```python
from build123d import *

# Parameters (mm, degrees)
CROQUIS1_W              = 210
CROQUIS1_H              = 50
CROQUIS1_R              = 2.5
CROQUIS1_R_2            = 2
SALIENTE_EXTRUIR1_DEPTH = 10
REDONDEO1_R             = 20


with BuildPart() as part:
    # Croquis1 → Saliente-Extruir1 (new body)
    with BuildSketch(Plane.XY):
        with Locations((105, -25)):
            Rectangle(CROQUIS1_W, CROQUIS1_H)
        with Locations((96, -28)):
            Circle(CROQUIS1_R, mode=Mode.SUBTRACT)
        Polygon((118, -27), (123, -27), (123, -32), (123, -37), (118, -37), (92, -37), (87, -37), (87, -32), (87, -27), (92, -27), (92, -32), (118, -32), align=None, mode=Mode.SUBTRACT)
        with Locations((114, -28)):
            Circle(CROQUIS1_R, mode=Mode.SUBTRACT)
        with Locations((4, -25)):
            Circle(CROQUIS1_R_2, mode=Mode.SUBTRACT)
        Polygon((67, -12), (76, -12), (76, -17), (67, -17), (67, -32), (76, -32), (76, -37), (67, -37), (61, -37), (61, -32), (61, -17), (61, -12), align=None, mode=Mode.SUBTRACT)
        Polygon((138, -12), (148, -12), (148, -17), (138, -17), (138, -21.5), (143, -21.5), (148, -21.5), (148, -26.5), (148, -31), (148, -36), (133, -36), (133, -31), (143, -31), (143, -26.5), (138, -26.5), (133, -26.5), (133, -21.5), (133, -17), (133, -12), align=None, mode=Mode.SUBTRACT)
        Polygon((87, -18), (87, -13), (92, -13), (102.5, -13), (102.5, -6), (107.5, -6), (107.5, -13), (118, -13), (123, -13), (123, -18), (123, -23), (118, -23), (118, -18), (107.5, -18), (102.5, -18), (92, -18), (92, -23), (87, -23), align=None, mode=Mode.SUBTRACT)
        with Locations((206, -25)):
            Circle(CROQUIS1_R_2, mode=Mode.SUBTRACT)
    extrude(amount=SALIENTE_EXTRUIR1_DEPTH)

    # Redondeo1
    redondeo1_edges = [part.edges().sort_by_distance(p)[0] for p in [
        (210, -50, 5),
        (0, -50, 5),
        (0, 0, 5),
        (210, 0, 5),
    ]]
    fillet(redondeo1_edges, radius=REDONDEO1_R)


solid = part.part
```
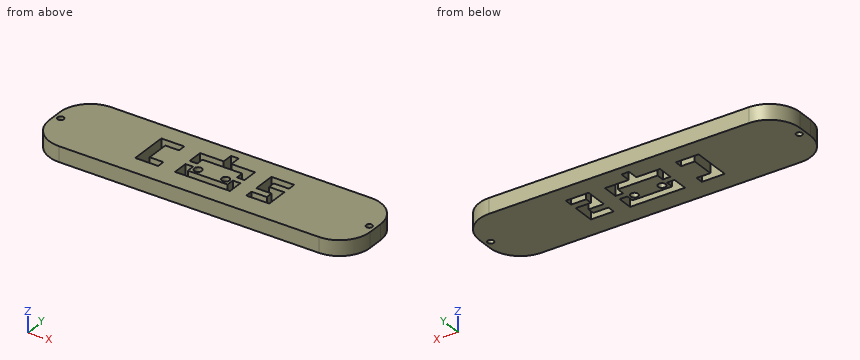
Can you work these out from the model? Positions are in its coordinate system, mm. Round coordinates to 2 decimals unless told otherwise and drop trailing zeros. Order: outer loops, then holes, each group sorted by start corner. A loop starts at its lowest first (then second) coordinate and runs counter-clockwise, first axis right, second up.
(1) If I drill on L1, parallel to Y at x = 119, z = 1; L2, parallel to Y at x = 96, z = 3; L3, parallel to X at y = -21, z = 1.5, over which ranges is the centre line in solid material (lowest first)?
Results are:
L1: y = -50 to -37, -27 to -23, -13 to 0
L2: y = -50 to -37, -32 to -30.5, -25.5 to -18, -13 to 0
L3: x = 0 to 61, 67 to 87, 92 to 118, 123 to 133, 138 to 210
(2) If we section it at D-D (y = -40): Please give me the cut outline in (x, z), plus the area to 3 significant figures.
Results are:
outline: (2.68, 0) - (207.32, 0) - (207.32, 10) - (2.68, 10) - close
area: 2,050 mm2
(3) If we section it at B-B (x = 206): Please give me the cut outline in (y, z).
Results are:
outline: (-42, 0) - (-27, 0) - (-27, 10) - (-42, 10) - close; (-23, 0) - (-8, 0) - (-8, 10) - (-23, 10) - close
(4) If we section it at C-C (z = 4): Count the separate pieces of the cut face and the enclosed holes in it, plus the area to 3 significant figures.
Results are:
separate pieces: 1
enclosed holes: 8
area: 9,090 mm2
(5) I'm going to push flat-ended pins straight in: pin 1 (1 mm diameter, centred on x = 123, y = -23.5, fed in from -Z); pin 2 (2.5 mm diameter, centred on y = -13.5, z = 5.5, fed in from -X); pin 3 (2.5 mm diameter, centred on y = -14, z = 4, fed in from -X); pin 4 (5 mm diameter, centred on y = -7.5, z = 5.5, fed in from +X). Where does each tip first touch, or does it pass through?
Results are:
pin 1: stops at z = 0
pin 2: stops at x = 0.7
pin 3: stops at x = 0.57
pin 4: stops at x = 207.32
(6) If we section it at A-A (x = 96): Please give me the cut outline in (y, z).
Results are:
outline: (-50, 0) - (-37, 0) - (-37, 10) - (-50, 10) - close; (-32, 0) - (-30.5, 0) - (-30.5, 10) - (-32, 10) - close; (-25.5, 0) - (-18, 0) - (-18, 10) - (-25.5, 10) - close; (-13, 0) - (0, 0) - (0, 10) - (-13, 10) - close
